from build123d import *

# Parameters (mm, degrees)
SKETCH_1_R          = 85.5
SKETCH_1_R_2        = 72.5
EXTRUDE_1_DEPTH     = 3
SKETCH_2_R          = 2.5
EXTRUDE_4_DEPTH     = 5
FILLET_1_R          = 1
SKETCH_3_R          = 2.65
CUT_EXTRUDE_1_DEPTH = 5


with BuildPart() as part:
    # 草图1 → 凸台-拉伸1 (new body)
    with BuildSketch(Plane(origin=(0, 0, 0), x_dir=(1, 0, 0), z_dir=(0, 1, 0))):
        with Locations(Location((0, 0, 0), (0, 0, 270))):
            Circle(SKETCH_1_R)
        with Locations(Location((0, 0, 0), (0, 0, 270))):
            Circle(SKETCH_1_R_2, mode=Mode.SUBTRACT)
    extrude(amount=EXTRUDE_1_DEPTH)

    # 草图2 → 凸台-拉伸4 (add)
    with BuildSketch(Plane(origin=(0, 3, 0), x_dir=(1, 0, 0), z_dir=(0, 1, 0))):
        with Locations(Location((0, 79, 0), (0, 0, 270))):
            Circle(SKETCH_2_R)
        with Locations(Location((79, 0, 0), (0, 0, 270))):
            Circle(SKETCH_2_R)
        with Locations(Location((0, -79, 0), (0, 0, 270))):
            Circle(SKETCH_2_R)
        with Locations(Location((-79, 0, 0), (0, 0, 270))):
            Circle(SKETCH_2_R)
    extrude(amount=EXTRUDE_4_DEPTH)

    # 圆角1
    fillet_1_edges = [part.edges().sort_by_distance(p)[0] for p in [
        (0, 3, -81.5),
        (-79, 3, -2.5),
        (79, 3, -2.5),
        (0, 3, 76.5),
    ]]
    fillet(fillet_1_edges, radius=FILLET_1_R)

    # 草图3 → 切除-拉伸1 (cut)
    with BuildSketch(Plane(origin=(0, 3, 0), x_dir=(1, 0, 0), z_dir=(0, 1, 0))):
        with Locations(Location((55.861435714, 55.861435714, 0), (0, 0, 270))):
            Circle(SKETCH_3_R)
        with Locations(Location((55.861435714, -55.861435714, 0), (0, 0, 270))):
            Circle(SKETCH_3_R)
        with Locations(Location((-55.861435714, -55.861435714, 0), (0, 0, 270))):
            Circle(SKETCH_3_R)
        with Locations(Location((-55.861435714, 55.861435714, 0), (0, 0, 270))):
            Circle(SKETCH_3_R)
    extrude(amount=-CUT_EXTRUDE_1_DEPTH, mode=Mode.SUBTRACT)


solid = part.part
Source: CAD feature listing. Evaluate the final solid. Frame: model axes, mm. A direction names the side the tool comes from. Coordinates: 2 decimals unless noted, no trailing zeros. Loops run counter-clockwise (first coordinate to the right, second up) from the corner with the lowest first, then second, coordinate; pieces in that order, holes last. Notation, with made-up numbers: (-32, 13.25) -> (-8, 13.25) arc R19 cw to (-8, 26.25) -> close; hole circle Ø9 at (43, -35). An arc over 180 degrees is marked (long way). Answer in a Markdown table with one row per item. Add a question column.
Q1. Pull-direction query (Z, two-part tool) for faces 1 (the face through (-53.234, 1.521, 55.516)), 2 (the face through (0.1, 6, -81.5)), 3 (the face through (19.4, 0, -70.1)), 4 (the face through (-76.52, 5.97, -0.33)); classes: pulls with the +Z half, pulls with the -Z half, needs draft (parallel to the pull), parting line crosses it, or undercut.
Q2. Reachability of faces 5 (the face through (0.1, 6, 76.5)), 6 (the face through (79, 8, 0)) from +Z, -Z, +X, -X, +Y, -Y: full face, straight path, thin tool, end or side. Return the list, or none.
Q3. Section D-D on z = 79. Return the cut outline in (x, y).
Q4. Section C-C on x = -79. Return the cut outline in (y, z), and give its area (3 significant figures).
Q5. Ray query, line 1 along X through (y, z) = (2, 0); line 2 along Z through (x, y) = (36.5, 2); line 3 along Y through (x, z) = (-60, -51). Return the intervals inside material, ascending.
Q6. Section B-B on z = 28.5. Return the cut outline in (x, y), and give its area (3 significant figures).
Q7. Section A-A on x = 0. Return the cut outline in (y, z).
Q8. Contact query for flat-ended pins moving along their axis: pin 1 Ø6 at (x, z) = (55.86, -55.86) entering from +Y; pin 2 Ø2 at (y, z) = (2.5, -42.5) entering from -X. Output: stop coordinate, or through.
Computed values:
| question | item | result |
|---|---|---|
| 1 | face 1 | undercut |
| 1 | face 2 | undercut |
| 1 | face 3 | needs draft |
| 1 | face 4 | parting line crosses it |
| 2 | face 5 | +Y |
| 2 | face 6 | +Z, -Z, +X, -X, +Y |
| 3 | outline | (-32.7, 0) -> (32.7, 0) -> (32.7, 3) -> (3.5, 3) arc R1 cw to (2.5, 4) -> (2.5, 8) -> (-2.5, 8) -> (-2.5, 4) arc R1 cw to (-3.5, 3) -> (-32.7, 3) -> close |
| 4 | outline | (0, -32.7) -> (3, -32.7) -> (3, -3.5) arc R1 cw to (4, -2.5) -> (8, -2.5) -> (8, 2.5) -> (4, 2.5) arc R1 cw to (3, 3.5) -> (3, 32.7) -> (0, 32.7) -> close |
| 4 | area | 222 mm^2 |
| 5 | line 1 | x = -85.5 to -72.5, 72.5 to 85.5 |
| 5 | line 2 | z = -77.32 to -62.64, 62.64 to 77.32 |
| 5 | line 3 | y = 0 to 3 |
| 6 | outline | (-80.61, 0) -> (-66.66, 0) -> (-66.66, 3) -> (-80.61, 3) -> close; (66.66, 0) -> (80.61, 0) -> (80.61, 3) -> (66.66, 3) -> close |
| 6 | area | 83.7 mm^2 |
| 7 | outline | (0, -85.5) -> (3, -85.5) -> (3, -82.5) arc R1 cw to (4, -81.5) -> (8, -81.5) -> (8, -76.5) -> (4, -76.5) arc R1 cw to (3, -75.5) -> (3, -72.5) -> (0, -72.5) -> close; (0, 72.5) -> (3, 72.5) -> (3, 75.5) arc R1 cw to (4, 76.5) -> (8, 76.5) -> (8, 81.5) -> (4, 81.5) arc R1 cw to (3, 82.5) -> (3, 85.5) -> (0, 85.5) -> close |
| 8 | pin 1 | stops at y = 3 |
| 8 | pin 2 | stops at x = -74.75 |
